Could you check a few things on this model? Use its own coordinates, in mm. Face numbers are marked on the shaded views. A direction names the side the tool comes from. Round coordinates to 2 decimals unless told otherwise and drop trailing zeros. Loops run counter-clockwise (first coordinate to the right, second up) from the corner with the lowest first, then second, coordinate; pieces in that order, holes last. Notation, with made-up numbers: (76.5, 52) -> (108.5, 52) arc R11 cw to (108.5, 58) -> close; hole circle Ø8 at (16, 9.25). An arc over 180 degrees is marked (long way). One line per item, written item: value.
```python
from build123d import *

# Parameters (mm, degrees)
SKETCH_1_R          = 10
EXTRUDE_1_DEPTH     = 2
SKETCH_2_R          = 3
SKETCH_2_R_2        = 1.5
CUT_EXTRUDE_1_DEPTH = 2
SKETCH_3_R          = 4.5
SKETCH_3_R_2        = 3
EXTRUDE_2_DEPTH     = 1


with BuildPart() as part:
    # 草图1 → 凸台-拉伸1 (new body)
    with BuildSketch(Plane(origin=(0, 0, 0), x_dir=(1, 0, 0), z_dir=(0, 1, 0))):
        Circle(SKETCH_1_R)
    extrude(amount=EXTRUDE_1_DEPTH)

    # 草图2 → 切除-拉伸1 (cut)
    with BuildSketch(Plane(origin=(0, 2, 0), x_dir=(1, 0, 0), z_dir=(0, 1, 0))):
        Circle(SKETCH_2_R)
        with Locations((0, 7)):
            Circle(SKETCH_2_R_2)
        with Locations((7, 0)):
            Circle(SKETCH_2_R_2)
        with Locations((0, -7)):
            Circle(SKETCH_2_R_2)
        with Locations((-7, 0)):
            Circle(SKETCH_2_R_2)
    extrude(amount=-CUT_EXTRUDE_1_DEPTH, mode=Mode.SUBTRACT)

    # 草图3 → 凸台-拉伸2 (add)
    with BuildSketch(Plane(origin=(0, 2, 0), x_dir=(1, 0, 0), z_dir=(0, 1, 0))):
        Circle(SKETCH_3_R)
        Circle(SKETCH_3_R_2, mode=Mode.SUBTRACT)
    extrude(amount=EXTRUDE_2_DEPTH)


solid = part.part
```
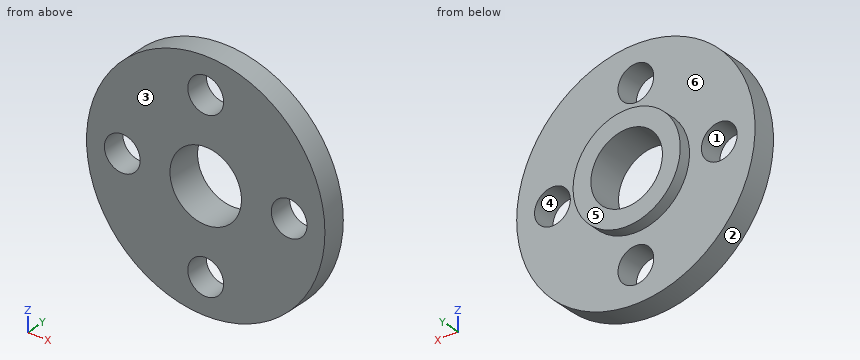
(1) We'd pull the mould along X, two halves only. Please class the marked faces 1, 2, 3 and 4: +X half, -X half, draft (parallel to the pull), parting line (faces both ways), or undercut.
Results below:
face 1: undercut
face 2: parting line
face 3: draft
face 4: undercut
(2) Imagine slicing it at A-A on x = 0. Write out the boundary of the cut face in (y, z).
Results below:
outline: (0, -10) -> (2, -10) -> (2, -8.5) -> (0, -8.5) -> close; (0, -5.5) -> (2, -5.5) -> (2, -4.5) -> (3, -4.5) -> (3, -3) -> (0, -3) -> close; (0, 3) -> (3, 3) -> (3, 4.5) -> (2, 4.5) -> (2, 5.5) -> (0, 5.5) -> close; (0, 8.5) -> (2, 8.5) -> (2, 10) -> (0, 10) -> close
(3) Imagine slicing it at B-B on z = 0. Write out the boundary of the cut face in (x, y), then the cut area to 3 significant figures.
Results below:
outline: (-10, 0) -> (-8.5, 0) -> (-8.5, 2) -> (-10, 2) -> close; (-5.5, 0) -> (-3, 0) -> (-3, 3) -> (-4.5, 3) -> (-4.5, 2) -> (-5.5, 2) -> close; (3, 0) -> (5.5, 0) -> (5.5, 2) -> (4.5, 2) -> (4.5, 3) -> (3, 3) -> close; (8.5, 0) -> (10, 0) -> (10, 2) -> (8.5, 2) -> close
area: 19.0 mm²
(4) On a 3-axis mill with a long thin cutter (end or side, diameter ignored), from which of +Z, -Z, +X, -X, +Y, -Y can I reach the whole of each face in a straight line? I mean the marked faces 5 and 6. Say none if no direction works.
Results below:
face 5: +Z, -Z, +X, -X, +Y
face 6: +Y
(5) Please list where these lines run through material, in increasing order: L1, parallel to X at y = 0.9, z = 0; L2, parallel to Y at x = -5, z = -0.5.
Results below:
L1: x = -10 to -8.5, -5.5 to -3, 3 to 5.5, 8.5 to 10
L2: y = 0 to 2
(6) For pin 1 Ø4 at (x, z) = (-7, 0) entering from +Y; pin 2 Ø1 at (y, z) = (0.5, -4.5) entering from +X, each with a flat end and sliding along its axis, tell me the tip position at first contact or that it passes through.
Results below:
pin 1: stops at y = 2
pin 2: stops at x = 9.17
(7) Imagine slicing it at C-C on y = 1.3. Write out the boundary of the cut face in (x, z).
Results below:
outline: circle Ø20 at (0, 0); hole circle Ø3 at (-7, 0); hole circle Ø6 at (0, 0); hole circle Ø3 at (0, -7); hole circle Ø3 at (0, 7); hole circle Ø3 at (7, 0)
(8) Imagine slicing it at D-D on z = 7. Write out the boundary of the cut face in (x, y), then the cut area to 3 significant figures.
Results below:
outline: (-7.14, 0) -> (-1.5, 0) -> (-1.5, 2) -> (-7.14, 2) -> close; (1.5, 0) -> (7.14, 0) -> (7.14, 2) -> (1.5, 2) -> close
area: 22.6 mm²
